Here's the drawing with two shaded views (mm, measured from the low corner). I have some questions. Coordinates: 2 decimals unless noted, no trailing zeros. Loops run counter-clockwise (first coordinate to the right, second up) from the corner with the lowest first, then second, coordinate; pieces in that order, holes last.
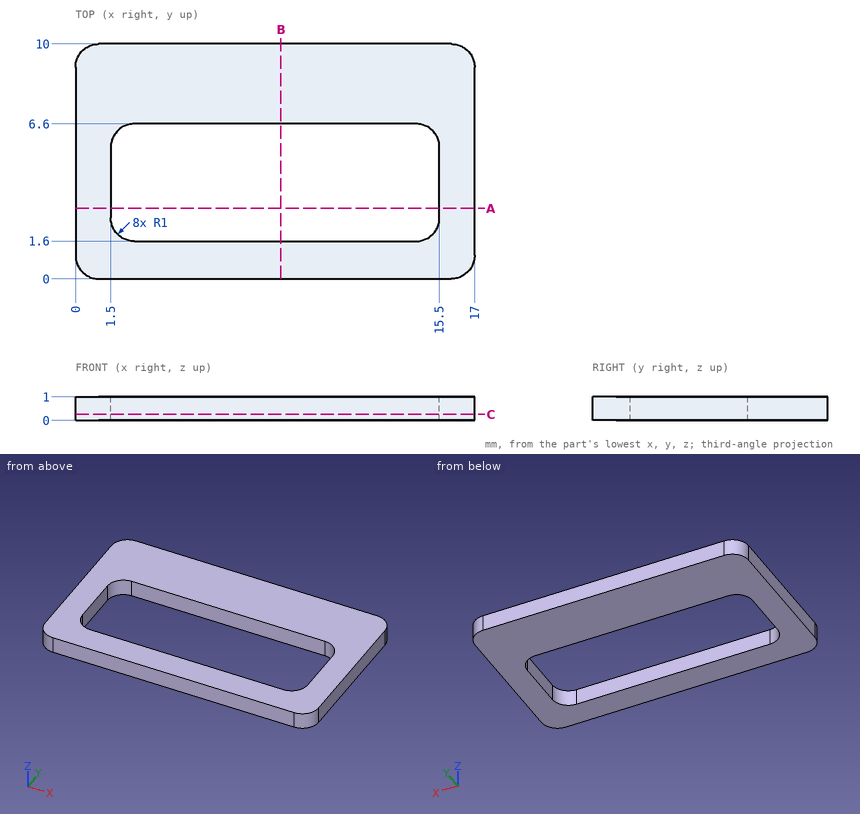
(1) I'm going to push flat-ended pins straight in: pin 1 (4 mm diameter, centred on x = 9.5, y = 4.5, fed in from +Z); pin 2 (3 mm diameter, centred on x = 4, y = 6, fed in from +Z). Where does each tip first touch, or does it pass through?
Check values:
pin 1: passes through
pin 2: stops at z = 1
(2) I want a section at A-A on y = 3. Write out the boundary of the cut face in (x, z).
Check values:
outline: (0, 0) - (1.5, 0) - (1.5, 1) - (0, 1) - close; (15.5, 0) - (17, 0) - (17, 1) - (15.5, 1) - close
(3) I want a section at C-C on z = 0.25. Write out the boundary of the cut face in (x, y), then the cut area to 3 significant figures.
Check values:
outline: (0, 1) arc R1 ccw to (1, 0) - (16, 0) arc R1 ccw to (17, 1) - (17, 9) arc R1 ccw to (16, 10) - (1, 10) arc R1 ccw to (0, 9) - close; hole (1.5, 2.6) arc R1 ccw to (2.5, 1.6) - (14.5, 1.6) arc R1 ccw to (15.5, 2.6) - (15.5, 5.6) arc R1 ccw to (14.5, 6.6) - (2.5, 6.6) arc R1 ccw to (1.5, 5.6) - close
area: 100 mm2
(4) I want a section at B-B on x = 8.75. Write out the boundary of the cut face in (y, z), then the cut area to 3 significant figures.
Check values:
outline: (0, 0) - (1.6, 0) - (1.6, 1) - (0, 1) - close; (6.6, 0) - (10, 0) - (10, 1) - (6.6, 1) - close
area: 5.00 mm2
(5) If I drill on probe 1 along X at (y, z) = (5, 0.2); probe 2 along Y at (x, z) = (11.25, 0.45); probe 3 along X at (y, z) = (6.25, 0.4), over which ranges is the centre line in solid material (lowest first)?
Check values:
probe 1: x = 0 to 1.5, 15.5 to 17
probe 2: y = 0 to 1.6, 6.6 to 10
probe 3: x = 0 to 1.74, 15.26 to 17
